```python
from build123d import *

# Parameters (mm, degrees)
SKETCH1_W           = 10
SKETCH1_H           = 7
REVOLVE1_ANGLE      = 180
SKETCH2_W           = 10
SKETCH2_H           = 7
BOSS_EXTRUDE1_DEPTH = 10
SKETCH4_W           = 10
SKETCH4_H           = 7
REVOLVE3_ANGLE      = 180
SKETCH5_R           = 1.25
CUT_EXTRUDE1_DEPTH  = 2.5


with BuildPart() as part:
    # Sketch1 → Revolve1 (revolve)
    with BuildSketch(Plane(origin=(0, 0, 0), x_dir=(0, 0, -1), z_dir=(1, 0, 0))):
        with Locations((0, 63.5)):
            Rectangle(SKETCH1_W, SKETCH1_H)
    revolve(axis=Axis((0, 0, 29.874383247), (0, 0, 1)), revolution_arc=REVOLVE1_ANGLE)

    # Sketch2 → Boss-Extrude1 (add)
    with BuildSketch(Plane(origin=(0, 0, 0), x_dir=(0, 0, -1), z_dir=(1, 0, 0))):
        with Locations((0, 63.5)):
            Rectangle(SKETCH2_W, SKETCH2_H)
        with Locations((0, -63.5)):
            Rectangle(SKETCH2_W, SKETCH2_H)
    extrude(amount=BOSS_EXTRUDE1_DEPTH)

    # Sketch4 → Revolve3 (revolve)
    with BuildSketch(Plane(origin=(10, 0, 0), x_dir=(0, 0, -1), z_dir=(1, 0, 0))):
        with Locations((0, 63.5)):
            Rectangle(SKETCH4_W, SKETCH4_H)
    revolve(axis=Axis((10, 0, 23.347655249), (0, 0, -1)), revolution_arc=REVOLVE3_ANGLE)

    # Sketch5 → Cut-Extrude1 (cut)
    with BuildSketch(Plane(origin=(0, -60, 0), x_dir=(1, 0, 0), z_dir=(0, 1, 0))):
        with Locations((5, 0)):
            Circle(SKETCH5_R)
    cut_extrude1 = extrude(amount=-CUT_EXTRUDE1_DEPTH, mode=Mode.SUBTRACT)

    # Mirror1: Cut-Extrude1 across plane
    add(cut_extrude1.mirror(Plane.ZX), mode=Mode.SUBTRACT)


solid = part.part
```
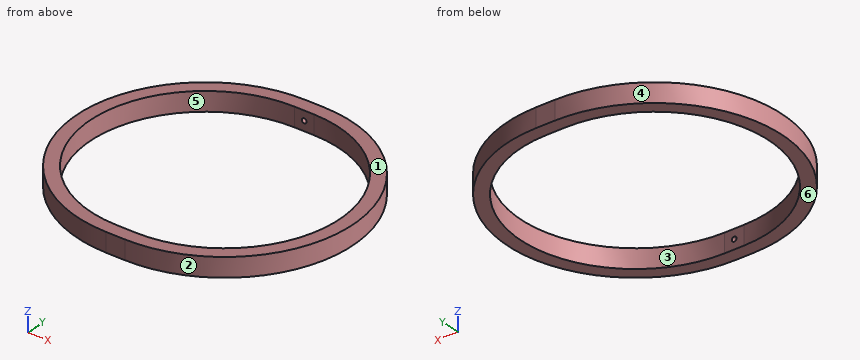
Geometry check sheet. Reference: the model listing, model coordinates, mm. Face numbers are marked on the shaded views. A direction names the side the tool comes from. Give positions to 0.01 mm unless a question says otherwise; leave off trailing zeros. Order: outer loops, then holes, each group sorted by start corner. A loop starts at its lowest first (then second) coordinate and runs counter-clockwise, first axis right, second up. Notation, with made-up numbers: (8.5, 53.5) - (40.5, 53.5) arc R22 ccw to (40.5, 60.5) - close; hole circle Ø7 at (64, -29.75). An arc over 180 degrees is marked (long way). Answer in a Markdown table with one row per item. Add a question column.
Q1. Material ranges on probe 1 along Z at (x, y) = (5, 60.95); probe 2 along Y at (x, z) = (6, 3.75); probe 3 along X at (y, z) = (50, -2), recorded low to high. Write a range as from..to.
Q2. Tool access check on the marked faces 5 and 6. Record the directions out of +Z, -Z, +X, -X, +Y, -Y that give a thin tool (end or side, any length) a straight path to the whole face; none if there is none.
Q3. Mould release check, pull along X, two halves, no side actions. Record for the marked faces 1, 2, 3 and 4: pulls with the +X half, pulls with the -X half, needs draft (parallel to the pull), parting line crosses it, or undercut.
Q4. Gauge pin test, flat ends, axial feed: pin 1 (1 mm diameter, centred on y = 29.5, z = -3.5, fed in from +X); pin 2 (3 mm diameter, centred on x = -4.5, z = -3.5, fed in from -Y); pin 3 (2 mm diameter, centred on y = -53, z = -2.5, fed in from -X). Record the tip position at first contact, or that the pin passes through.
Q5. Cross-section at C-C, the plane z = -2.75. Enter the section's corners in (x, y).
Q6. Cross-section at A-A, the plane x = -45. Enter the section's corners in (y, z).
Q7. Cross-section at B-B, the plane y = 48. Enter the section's corners in (x, z), then the cut area to 3 significant figures.
Check values:
| question | item | result |
|---|---|---|
| 1 | probe 1 | z = -5..-1.25, 1.25..5 |
| 1 | probe 2 | y = -67..-60, 60..67 |
| 1 | probe 3 | x = -44.6..-33.17, 43.17..54.6 |
| 2 | face 5 | +Z, -Z |
| 2 | face 6 | -Z, +X, -X, +Y, -Y |
| 3 | face 1 | needs draft |
| 3 | face 2 | pulls with the +X half |
| 3 | face 3 | undercut |
| 3 | face 4 | pulls with the -X half |
| 4 | pin 1 | stops at x = 70.4 |
| 4 | pin 2 | stops at y = -66.93 |
| 4 | pin 3 | stops at x = -42.25 |
| 5 | outline | (0, -67) - (10, -67) arc R67 ccw to (10, 67) - (0, 67) arc R67 ccw to start; hole (0, -60) - (10, -60) arc R60 ccw to (10, 60) - (0, 60) arc R60 ccw to start |
| 6 | outline | (-49.64, -5) - (-39.69, -5) - (-39.69, 5) - (-49.64, 5) - close; (39.69, -5) - (49.64, -5) - (49.64, 5) - (39.69, 5) - close |
| 7 | outline | (-46.74, -5) - (-36, -5) - (-36, 5) - (-46.74, 5) - close; (46, -5) - (56.74, -5) - (56.74, 5) - (46, 5) - close |
| 7 | area | 215 mm^2 |
